Part model, mm, in its own coordinate system. A direction names the side the tool comes from. Give positions to 0.01 mm unless a question says otherwise; leave off trailing zeros. Write each loop counter-clockwise with the first axis right and the second up, starting at its lowest first coordinate (ties: lowest second). Pieces come first, ordered by that corner, then holes.
from build123d import *

# Parameters (mm, degrees)
BOSS_EXTRUDE2_DEPTH   = 40
BOSS_EXTRUDE3_DEPTH   = 80
SKETCH5_R             = 4.125
CUT_EXTRUDE1_DEPTH    = 43
CHAMFER1_SIZE         = 0.5
CHAMFER1_SIZE2        = 0.866025404
CHAMFER1_PART_2_SIZE  = 0.5
CHAMFER1_PART_2_SIZE2 = 0.866025404
CHAMFER1_PART_3_SIZE  = 0.5
CHAMFER1_PART_3_SIZE2 = 0.866025404
CHAMFER1_PART_4_SIZE  = 0.5
CHAMFER1_PART_4_SIZE2 = 0.866025404


with BuildPart() as part:
    # Sketch2 → Boss-Extrude2 (new body)
    with BuildSketch(Plane(origin=(0, 0, 0), x_dir=(1, 0, 0), z_dir=(0, 1, 0))):
        Polygon((-31.312103746, 30), (-31.312103746, 0), (48.687896254, 0), (48.687896254, 30), (28.787896254, 30), (28.787896254, 10.4), (-11.412103746, 10.4), (-11.412103746, 30), align=None)
    extrude(amount=BOSS_EXTRUDE2_DEPTH)

    # Sketch4 → Boss-Extrude3 (add)
    with BuildSketch(Plane(origin=(48.687896254, 0, 0), x_dir=(0, 0, -1), z_dir=(1, 0, 0))):
        Polygon((0, 0), (-12, 0), (-12, 14.9), (-2, 14.9), (-2, 25.1), (-12, 25.1), (-12, 40), (0, 40), align=None)
    extrude(amount=-BOSS_EXTRUDE3_DEPTH)

    # Sketch5 → Cut-Extrude1 (cut, through all)
    with BuildSketch(Plane.XY.offset(12)):
        with Locations((-3.812103746, 31.5)):
            Circle(SKETCH5_R)
        with Locations((21.187896254, 31.5)):
            Circle(SKETCH5_R)
        with Locations((21.187896254, 8.5)):
            Circle(SKETCH5_R)
        with Locations((-3.812103746, 8.5)):
            Circle(SKETCH5_R)
        with Locations((-21.312103746, 31.5)):
            Circle(SKETCH5_R)
        with Locations((-21.312103746, 8.5)):
            Circle(SKETCH5_R)
        with Locations((38.687896254, 8.5)):
            Circle(SKETCH5_R)
        with Locations((38.687896254, 31.5)):
            Circle(SKETCH5_R)
        with Locations((8.687896254, 20)):
            Circle(SKETCH5_R)
    extrude(amount=-CUT_EXTRUDE1_DEPTH, mode=Mode.SUBTRACT)

    # Chamfer1
    chamfer1_edges = [part.edges().sort_by_distance(p)[0] for p in [
        (8.687896254, 14.9, 12),
        (34.562896254, 8.5, 12),
        (-25.437103746, 8.5, 12),
        (-7.937103746, 8.5, 12),
        (17.062896254, 8.5, 12),
    ]]
    chamfer1_side = [part.faces().sort_by_distance(p)[0] for p in [
        (8.687896254, 7.220474811, 12),
    ]]
    chamfer(chamfer1_edges, length=CHAMFER1_SIZE, length2=CHAMFER1_SIZE2, reference=chamfer1_side[0])

    # Chamfer1 part 2
    chamfer1_part_2_edges = [part.edges().sort_by_distance(p)[0] for p in [
        (8.687896254, 25.1, 12),
    ]]
    chamfer1_part_2_side = [part.faces().sort_by_distance(p)[0] for p in [
        (8.687896254, 25.1, 7),
    ]]
    chamfer(chamfer1_part_2_edges, length=CHAMFER1_PART_2_SIZE, length2=CHAMFER1_PART_2_SIZE2, reference=chamfer1_part_2_side[0])

    # Chamfer1 part 3
    chamfer1_part_3_edges = [part.edges().sort_by_distance(p)[0] for p in [
        (-7.937103746, 31.5, 12),
        (34.562896254, 31.5, 12),
        (-25.437103746, 31.5, 12),
        (17.062896254, 31.5, 12),
    ]]
    chamfer1_part_3_side = [part.faces().sort_by_distance(p)[0] for p in [
        (8.687896254, 32.779525189, 12),
    ]]
    chamfer(chamfer1_part_3_edges, length=CHAMFER1_PART_3_SIZE, length2=CHAMFER1_PART_3_SIZE2, reference=chamfer1_part_3_side[0])

    # Chamfer1 part 4
    chamfer1_part_4_edges = [part.edges().sort_by_distance(p)[0] for p in [
        (4.562896254, 20, 2),
    ]]
    chamfer1_part_4_side = [part.faces().sort_by_distance(p)[0] for p in [
        (8.687896254, 15.706476286, 2),
    ]]
    chamfer(chamfer1_part_4_edges, length=CHAMFER1_PART_4_SIZE, length2=CHAMFER1_PART_4_SIZE2, reference=chamfer1_part_4_side[0])


solid = part.part
1) 3-axis set-ups, long thin cutter, end or side, ignore diameter. For faces 1 (the flat face through (9, 25.1, 7)), 2 (the flat face through (39, 20, -30)): which of +Z, -Z, +X, -X, +Y, -Y reach the whole face in a straight line?
Check result:
face 1: +Z, +X, -X
face 2: -Z, +X, -X, +Y, -Y
2) Saw through at A-A (y = 31.5). State how many separate pieces and enclosed holes the cut face has, and give its area (3 significant figures).
Check result:
separate pieces: 5
enclosed holes: 0
area: 1,510 mm2
3) Saw through at B-B (y = 20). Write the cut outline in (x, z), and give its area (3 significant figures).
Check result:
outline: (-31.31, -30) - (-11.41, -30) - (-11.41, -10.4) - (4.56, -10.4) - (4.56, 1.13) - (4.06, 2) - (-31.31, 2) - close; (12.81, -10.4) - (28.79, -10.4) - (28.79, -30) - (48.69, -30) - (48.69, 2) - (13.31, 2) - (12.81, 1.13) - close
area: 1,670 mm2
4) Drill centre lines: L1, parallel to Y at x = -4, z = -6.5; L2, parallel to Y at x = 9, z = 7; L3, parallel to X at y = 31, z = 5. Where is each one in solid material? Low to high.
Check result:
L1: y = 0 to 4.38, 12.62 to 27.38, 35.62 to 40
L2: y = 0 to 14.9, 25.1 to 40
L3: x = -31.31 to -25.41, -17.22 to -7.91, 0.28 to 17.09, 25.28 to 34.59, 42.78 to 48.69
5) Flat gauge pins, fed straight in: P1, Ø1, axis at x = -8, y = 31.5, coming from the -Z side; P2, Ø8, axis at x = 28, y = 21.5, coming from the +Z side; P3, Ø10.5, axis at x = 8.69, y = 20, coming from the +Z side. Where does each tip first touch, or does it go through?
Check result:
P1: stops at z = -10.4
P2: stops at z = 11.73
P3: stops at z = 11.59
6) Mould opens along Y. For faces 3 (the flat face through (9, 40, -4)), 4 (the flat face through (9, 15, -10.4)), 5 (the cylindrical face through (-24.35, 34.29, -9.15)) say: +Y half, -Y half, draft (parallel to the pull), parting line (faces both ways), or undercut.
Check result:
face 3: +Y half
face 4: draft
face 5: undercut
